Check sheet for the modelled part. Datum: model origin and axes. Units: mm. Face numbers are marked on the shaded views. A direction names the side the tool comes from. Give positions to 0.01 mm unless a question says otherwise; leave off trailing zeros. Write each loop counter-clockwise with the first axis right and the second up, starting at its lowest first coordinate (ties: lowest second). Pieces come first, ordered by that corner, then holes. Notation, with made-up numbers: (-18.75, -9.75) - (17.25, -9.75) arc R23 cw to (17.25, -0.75) - close; hole circle Ø1 at (15.5, 82). An arc over 180 degrees is marked (long way). Return JSON: item names as keys, results as strings. Group by question number.
Autodesk Inventor part; units mm, degrees
ref_plane "YZ Plane" through (0, 0, 0) normal (1, 0, 0) x (0, 1, 0)
ref_plane "XZ Plane" through (0, 0, 0) normal (0, 1, 0) x (-1, 0, 0)
ref_plane "XY Plane" through (0, 0, 0) normal (0, 0, 1) x (1, 0, 0)
sketch "Sketch1" plane through (0, 0, 0) normal (0, 1, 0) x (-1, 0, 0)
  line L0 (37.5, 82.5) -> (-37.5, 82.5)
  line L1 (-37.5, 82.5) -> (-37.5, -82.5)
  line L2 (-37.5, -82.5) -> (37.5, -82.5)
  line L3 (37.5, -82.5) -> (37.5, 82.5)
  point P0 (0, 0)
  point P1 (37.5, 0)
  point P2 (0, -82.5)
  dimension "d0" = 75
  dimension "d1" = 165
extrude "Extrusion1" add sketch "Sketch1" along normal blind 38.1
sketch "Sketch2" plane through (0, 38.1, 0) normal (0, 1, 0) x (1, 0, 0)
  line L0 (-33.69, -78.69) -> (33.69, -78.69)
  line L1 (33.69, -78.69) -> (33.69, 78.69)
  line L2 (33.69, 78.69) -> (-33.69, 78.69)
  line L3 (-33.69, 78.69) -> (-33.69, -78.69)
  line L4 (-37.5, 82.5) -> (-37.5, -82.5)
  line L5 (37.5, 82.5) -> (-37.5, 82.5)
  line L6 (37.5, -82.5) -> (37.5, 82.5)
  line L7 (-37.5, -82.5) -> (37.5, -82.5)
  point P0 (0, 0)
  dimension "d4" = 3.81
  dimension "d5" = 3.81
  dimension "d6" = 3.81
  dimension "d7" = 3.81
extrude "Extrusion2" cut sketch "Sketch2" against normal blind 34.925 contours L3 L2 L1 L0
sketch "Sketch3" plane through (0, 38.1, 0) normal (0, 1, 0) x (1, 0, 0)
  line L0 (-36.611, -46.482) -> (-36.611, -31.242)
  line L1 (-36.611, -31.242) -> (-34.452, -31.242)
  line L2 (-34.452, -31.242) -> (-34.452, -46.482)
  line L3 (-34.452, -46.482) -> (-36.611, -46.482)
  line L4 (-36.611, 31.242) -> (-36.611, 46.482)
  line L5 (-36.611, 46.482) -> (-34.452, 46.482)
  line L6 (-34.452, 46.482) -> (-34.452, 31.242)
  line L7 (-34.452, 31.242) -> (-36.611, 31.242)
  line L8 (-36.611, -7.62) -> (-36.611, 7.62)
  line L9 (-36.611, 7.62) -> (-34.452, 7.62)
  line L10 (-34.452, 7.62) -> (-34.452, -7.62)
  line L11 (-34.452, -7.62) -> (-36.611, -7.62)
  line L12 (-33.69, -78.69) -> (-33.69, 78.69)
  line L13 (0, -72.064) -> (0, 82.0809)
  line L14 (36.611, 46.482) -> (34.452, 46.482)
  line L15 (36.611, 7.62) -> (34.452, 7.62)
  line L16 (34.452, 7.62) -> (34.452, -7.62)
  line L17 (36.611, -7.62) -> (36.611, 7.62)
  line L18 (34.452, -7.62) -> (36.611, -7.62)
  line L19 (36.611, -46.482) -> (36.611, -31.242)
  line L20 (36.611, -31.242) -> (34.452, -31.242)
  line L21 (34.452, -31.242) -> (34.452, -46.482)
  line L22 (34.452, -46.482) -> (36.611, -46.482)
  line L23 (36.611, 31.242) -> (36.611, 46.482)
  line L24 (34.452, 46.482) -> (34.452, 31.242)
  line L25 (34.452, 31.242) -> (36.611, 31.242)
  point P0 (0, 0)
  point P1 (-35.5315, -31.242)
  point P2 (-35.5315, 31.242)
  point P3 (-35.5315, -7.62)
  point P4 (-35.5315, 7.62)
  point P5 (-34.452, 0)
  dimension "d10" = 2.159
  dimension "d11" = 2.159
  dimension "d12" = 2.159
  dimension "d13" = 23.622
  dimension "d14" = 23.622
  dimension "d15" = 15.24
  dimension "d16" = 15.24
  dimension "d17" = 15.24
  dimension "d18" = 0.762
  dimension "d19" = 0.762
  dimension "d20" = 0.762
extrude "Extrusion3" add sketch "Sketch3" along normal blind 5.08
sketch "Sketch12" plane through (-37.5, 0, -82.5) normal (-1, 0, 0) x (0, 0, 1)
  line L0 (5.08, 36.83) -> (26.0858, 36.83)
  line L1 (26.0858, 36.83) -> (26.0858, 22.098)
  line L2 (26.0858, 22.098) -> (5.08, 22.098)
  line L3 (5.08, 22.098) -> (5.08, 36.83)
  line L4 (0, 0) -> (0, 38.1)
  line L5 (0, 38.1) -> (165, 38.1)
  point P0 (82.5, 0)
  dimension "d85" = 14.732
  dimension "d86" = 21.0058
  dimension "d87" = 5.08
  dimension "d88" = 1.27
extrude "Extrusion10" cut sketch "Sketch12" against normal blind 13.0937
sketch "Sketch13" plane through (0, 3.175, 0) normal (0, 1, 0) x (1, 0, 0)
  line L0 (-33.69, 78.69) -> (33.69, 78.69)
  line L1 (-33.69, 78.69) -> (26.31, 78.69)
  line L2 (33.69, -71.31) -> (-26.31, -71.31)
  line L3 (-26.31, -71.31) -> (-26.31, 78.69)
  line L4 (-26.31, 78.69) -> (33.69, 78.69)
  line L5 (33.69, 78.69) -> (33.69, -71.31)
  line L6 (33.69, 78.69) -> (33.69, -78.69)
  point P0 (0, 0)
  point P1 (33.69, 3.69)
  point P2 (33.69, 0)
  dimension "d93" = 150
  dimension "d94" = 60
extrude "Extrusion11" add sketch "Sketch13" along normal blind 2.54
sketch "Sketch14" plane through (0, 5.715, 0) normal (0, 1, 0) x (1, 0, 0)
  circle A0 centre (-16.3328, 52.2995) radius 1.27
  circle A1 centre (21.5397, 52.2995) radius 1.27
  circle A2 centre (-16.3328, -48.2599) radius 1.27
  circle A3 centre (21.5397, -48.2599) radius 1.27
  line L0 (-33.69, 78.69) -> (33.69, 78.69)
  point P0 (0, 0)
  dimension "d97" = 2.54
  dimension "d98" = 2.54
  dimension "d99" = 2.54
  dimension "d100" = 2.54
  dimension "d101" = 26.3905
sketch "Sketch15" plane through (37.5, 0, -82.5) normal (0, 0, -1) x (-1, 0, 0)
  line L0 (21, 18) -> (33, 18)
  line L1 (33, 18) -> (33, 25)
  line L2 (33, 25) -> (21, 25)
  line L3 (21, 25) -> (21, 18)
  line L4 (0, 0) -> (0, 38.1)
  line L5 (0, 0) -> (75, 0)
  line L6 (0, 38.1) -> (75, 38.1)
  point P0 (37.5, 0)
  point P1 (27, 25)
  dimension "d104" = 12
  dimension "d105" = 7
  dimension "d120" = 21
  dimension "d121" = 18
extrude "Extrusion12" cut sketch "Sketch15" against normal blind 39.0525
sketch "Sketch16" plane through (0, 5.715, 0) normal (0, 1, 0) x (1, 0, 0)
  circle A0 centre (28.69, -66.31) radius 1.27
  circle A1 centre (-21.31, -66.31) radius 1.27
  circle A2 centre (28.69, 73.69) radius 1.27
  circle A3 centre (-21.31, 73.69) radius 1.27
  line L0 (33.69, 78.69) -> (33.69, -78.69)
  line L1 (-33.69, 78.69) -> (33.69, 78.69)
  line L2 (-26.31, 78.69) -> (-26.31, -71.31)
  line L3 (-26.31, -71.31) -> (33.69, -71.31)
  point P0 (0, 0)
  dimension "d108" = 2.54
  dimension "d109" = 5
  dimension "d110" = 5
  dimension "d111" = 5
  dimension "d112" = 5
  dimension "d113" = 5
  dimension "d114" = 5
  dimension "d115" = 5
  dimension "d116" = 5
  dimension "d122" = 2.54
extrude "Extrusion13" cut sketch "Sketch16" against normal blind 4.7625 contours A0 | A1 | A2 | A3
properties part number "tapaderaf"
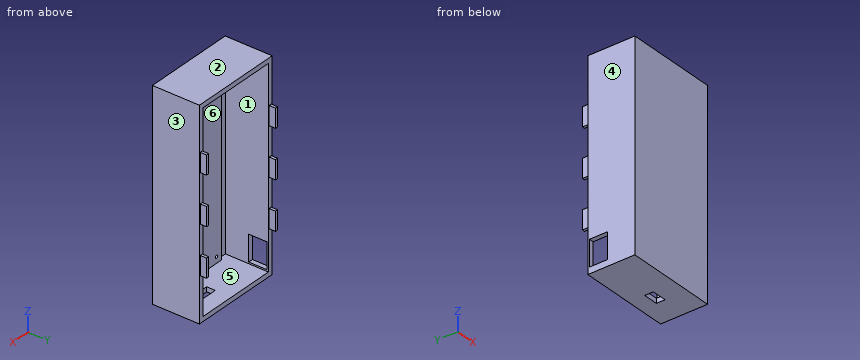
Item 1: Access from +Z, -Z, +X, -X, +Y, -Y to the whole of each face (thin tool, end or side, straight path). Record for the marked faces 1 and 2.
Item 2: Material ranges on line 1 along Z through (x, y) = (28.69, 2.3); line 2 along Z through (x, y) = (28.69, 3.95); line 3 along X through (y, z) = (34.5, 6.5), recorded low to high. Write a range as from..to.
Item 3: Depth check by flat-ended pin: pin 1 (4 mm diameter, centred on y = 41, z = 38, fed in from +X); pin 2 (5 mm diameter, centred on x = 5, z = 14, fed in from +Y) (3 decimals); pin 3 (3.5 mm diameter, centred on x = -21.31, z = 66.31, fed in from -Y); pin 4 (2.5 mm diameter, centred on y = 39.5, z = 42.5, fed in from -X). Enter the tip coordinate at first touch or a pass-through.
Item 4: Section check D-D on y = 31.5. Record the cut outline in (x, z).
Item 5: Section check A-A on y = 12. Record the cut outline in (x, z).
Item 6: Mould release check, pull along X, two halves, no side actions. Record for the marked faces 3, 4, 5 and 6: +X half, -X half, draft (parallel to the pull), parting line (faces both ways), or undercut.
Item 7: Section check B-B on x = -29. Record the cut outline in (y, z) (3 decimals).
Item 8: Section check C-C on z = -33.5. Record the cut outline in (x, y) (3 decimals).
Reply:
{
 "1": {"face 1": "+Y", "face 2": "+Z, +X, -X, +Y, -Y"},
 "2": {"line 1": "-82.5..-74.96, -72.42..65.04, 67.58..82.5", "line 2": "-82.5..-74.96, -72.42..65.04, 67.58..71.31, 78.69..82.5", "line 3": "-37.5..-33.69, 33.69..37.5"},
 "3": {"pin 1": "x = 36.61", "pin 2": "y = 5.715", "pin 3": "y = 0", "pin 4": "x = -36.61"},
 "4": {"outline": "(-37.5, -82.5) - (37.5, -82.5) - (37.5, 82.5) - (-37.5, 82.5) - (-37.5, -56.41) - (-33.69, -56.41) - (-33.69, 78.69) - (33.69, 78.69) - (33.69, -78.69) - (-33.69, -78.69) - (-33.69, -77.42) - (-37.5, -77.42) - close"},
 "5": {"outline": "(-37.5, -82.5) - (37.5, -82.5) - (37.5, 82.5) - (-37.5, 82.5) - close; hole (-33.69, -78.69) - (33.69, -78.69) - (33.69, 78.69) - (-33.69, 78.69) - close"},
 "6": {"face 3": "+X half", "face 4": "-X half", "face 5": "undercut", "face 6": "undercut"},
 "7": {"outline": "(0, -82.5) - (38.1, -82.5) - (38.1, -78.69) - (3.175, -78.69) - (3.175, 78.69) - (38.1, 78.69) - (38.1, 82.5) - (0, 82.5) - close"},
 "8": {"outline": "(-37.5, 0) - (37.5, 0) - (37.5, 38.1) - (36.611, 38.1) - (36.611, 43.18) - (34.452, 43.18) - (34.452, 38.1) - (33.69, 38.1) - (33.69, 5.715) - (-26.31, 5.715) - (-26.31, 3.175) - (-33.69, 3.175) - (-33.69, 38.1) - (-34.452, 38.1) - (-34.452, 43.18) - (-36.611, 43.18) - (-36.611, 38.1) - (-37.5, 38.1) - close"}
}
